from build123d import *

# Parameters (mm, degrees)
BOSS_EXTRUDE1_DEPTH   = 1.57
BOSS_EXTRUDE1_2_DEPTH = 1.57
SKETCH2_W             = 20.9
SKETCH2_H             = 15.9
SKETCH2_W_2           = 94.45
SKETCH2_H_2           = 0.025
SKETCH2_H_3           = 6.025
BOSS_EXTRUDE3_DEPTH   = 6


with BuildPart() as part:
    # Sketch1 → Boss-Extrude1 (new body)
    with BuildSketch(Plane.XY.offset(7.67)):
        with BuildLine():
            Line((-10.2, 60.925), (-45.45, 60.925))
            Line((-45.45, 60.925), (-45.45, 66.925))
            Line((-45.45, 66.925), (45.45, 66.925))
            Line((45.45, 66.925), (45.45, 60.925))
            Line((45.45, 60.925), (10.2, 60.925))
            ThreePointArc((10.2, 60.925), (9.369149532, 61.269149532), (9.025, 62.1))
            Line((9.025, 62.1), (9.025, 63.7))
            ThreePointArc((9.025, 63.7), (8.666205807, 64.566205807), (7.8, 64.925))
            Line((7.8, 64.925), (6.2, 64.925))
            ThreePointArc((6.2, 64.925), (5.333794193, 64.566205807), (4.975, 63.7))
            Line((4.975, 63.7), (4.975, 62.1))
            ThreePointArc((4.975, 62.1), (4.630850468, 61.269149532), (3.8, 60.925))
            Line((3.8, 60.925), (-3.8, 60.925))
            ThreePointArc((-3.8, 60.925), (-4.630850468, 61.269149532), (-4.975, 62.1))
            Line((-4.975, 62.1), (-4.975, 63.7))
            ThreePointArc((-4.975, 63.7), (-5.333794193, 64.566205807), (-6.2, 64.925))
            Line((-6.2, 64.925), (-7.8, 64.925))
            ThreePointArc((-7.8, 64.925), (-8.666205807, 64.566205807), (-9.025, 63.7))
            Line((-9.025, 63.7), (-9.025, 62.1))
            ThreePointArc((-9.025, 62.1), (-9.369149532, 61.269149532), (-10.2, 60.925))
        make_face()
    extrude(amount=-BOSS_EXTRUDE1_DEPTH)



with BuildPart() as body_2:
    # Sketch1 → Boss-Extrude1 2 (new body)
    with BuildSketch(Plane.XY.offset(7.67)):
        with BuildLine():
            Line((10.2, -60.925), (45.45, -60.925))
            Line((45.45, -60.925), (45.45, -66.925))
            Line((45.45, -66.925), (-45.45, -66.925))
            Line((-45.45, -66.925), (-45.45, -60.925))
            Line((-45.45, -60.925), (-10.2, -60.925))
            ThreePointArc((-10.2, -60.925), (-9.369149532, -61.269149532), (-9.025, -62.1))
            Line((-9.025, -62.1), (-9.025, -63.7))
            ThreePointArc((-9.025, -63.7), (-8.666205807, -64.566205807), (-7.8, -64.925))
            Line((-7.8, -64.925), (-6.2, -64.925))
            ThreePointArc((-6.2, -64.925), (-5.333794193, -64.566205807), (-4.975, -63.7))
            Line((-4.975, -63.7), (-4.975, -62.1))
            ThreePointArc((-4.975, -62.1), (-4.630850468, -61.269149532), (-3.8, -60.925))
            Line((-3.8, -60.925), (3.8, -60.925))
            ThreePointArc((3.8, -60.925), (4.630850468, -61.269149532), (4.975, -62.1))
            Line((4.975, -62.1), (4.975, -63.7))
            ThreePointArc((4.975, -63.7), (5.333794193, -64.566205807), (6.2, -64.925))
            Line((6.2, -64.925), (7.8, -64.925))
            ThreePointArc((7.8, -64.925), (8.666205807, -64.566205807), (9.025, -63.7))
            Line((9.025, -63.7), (9.025, -62.1))
            ThreePointArc((9.025, -62.1), (9.369149532, -61.269149532), (10.2, -60.925))
        make_face()
    extrude(amount=-BOSS_EXTRUDE1_2_DEPTH)


with BuildPart() as part_1:
    add(part.part)

    add(body_2.part)  # Boss-Extrude3 merges body 2
    # Sketch2 → Boss-Extrude3 (add)
    with BuildSketch(Plane.XY.offset(0.1)):
        with BuildLine():
            ThreePointArc((-45.621153846, 16.138909297), (-42.65479168, 19.145865857), (-41.280343138, 23.139859279))
            ThreePointArc((-41.280343138, 23.139859279), (-44.331790058, 26.826513587), (-45.425, 31.485659466))
            Line((-45.425, 31.485659466), (-45.45, 66.925))
            Line((-45.45, 66.925), (45.45, 66.925))
            Line((45.45, 66.925), (45.425, 31.485659466))
            ThreePointArc((45.425, 31.485659466), (44.331790058, 26.826513587), (41.280343138, 23.139859279))
            ThreePointArc((41.280343138, 23.139859279), (42.65479168, 19.145865857), (45.621153846, 16.138909297))
            ThreePointArc((45.621153846, 16.138909297), (46.797776617, 14.880036243), (47.225, 13.21070024))
            Line((47.225, 13.21070024), (47.225, 0.025))
            Line((47.225, 0.025), (-47.225, 0.025))
            Line((-47.225, 0.025), (-47.225, 13.21070024))
            ThreePointArc((-47.225, 13.21070024), (-46.797776617, 14.880036243), (-45.621153846, 16.138909297))
        make_face()
        with Locations((0, 52.95)):
            Rectangle(SKETCH2_W, SKETCH2_H, mode=Mode.SUBTRACT)
        with Locations((0, 0.0125)):
            Rectangle(SKETCH2_W_2, SKETCH2_H_2)
        with Locations((0, -0.0125)):
            Rectangle(SKETCH2_W_2, SKETCH2_H_2)
        with BuildLine():
            Line((-47.225, -0.025), (-47.225, -13.21070024))
            ThreePointArc((-47.225, -13.21070024), (-46.797776617, -14.880036243), (-45.621153846, -16.138909297))
            ThreePointArc((-45.621153846, -16.138909297), (-42.65479168, -19.145865857), (-41.280343138, -23.139859279))
            ThreePointArc((-41.280343138, -23.139859279), (-44.331790058, -26.826513587), (-45.425, -31.485659466))
            Line((-45.425, -31.485659466), (-45.45, -66.925))
            Line((-45.45, -66.925), (-30.45, -66.925))
            Line((-30.45, -66.925), (-30.45, -45))
            Line((-30.45, -45), (-10.45, -45))
            Line((-10.45, -45), (10.45, -45))
            Line((10.45, -45), (30.45, -45))
            Line((30.45, -45), (30.45, -66.925))
            Line((30.45, -66.925), (45.45, -66.925))
            Line((45.45, -66.925), (45.425, -31.485659466))
            ThreePointArc((45.425, -31.485659466), (44.331790058, -26.826513587), (41.280343138, -23.139859279))
            ThreePointArc((41.280343138, -23.139859279), (42.65479168, -19.145865857), (45.621153846, -16.138909297))
            ThreePointArc((45.621153846, -16.138909297), (46.797776617, -14.880036243), (47.225, -13.21070024))
            Line((47.225, -13.21070024), (47.225, -0.025))
            Line((47.225, -0.025), (-47.225, -0.025))
        make_face()
        Polygon((10.45, -60.9), (10.45, -66.925), (30.45, -66.925), (30.45, -45), (10.45, -45), align=None)
        Polygon((-30.45, -45), (-30.45, -66.925), (-10.45, -66.925), (-10.45, -60.9), (-10.45, -45), align=None)
        with Locations((0, -63.9125)):
            Rectangle(SKETCH2_W, SKETCH2_H_3)
    extrude(amount=BOSS_EXTRUDE3_DEPTH)


solid = part_1.part
Here's how the part is built. I have some questions about the finished solid (model axes, mm). A direction names the side the tool comes from. Coordinates: 2 decimals unless noted, no trailing zeros. Loops run counter-clockwise (first coordinate to the right, second up) from the corner with the lowest first, then second, coordinate; pieces in that order, holes last. Notation, with made-up numbers: (32.25, 16) -> (44.25, 16) arc R30 ccw to (44.25, 43) -> close; hole circle Ø2 at (-23.5, 35). An arc over 180 degrees is marked (long way). Use one line per item in the form item = value. Start each with the question number.
(1) If we section it at A-A (z = 2.5): Please give me the cut outline in (x, y) (3 decimals), then the cut area to 3 significant figures.
(2) Will these pins go through, and if not, where does the flat tip stop? pin 1 (0.8 mm diameter, centred on y = 62.5, z = 7, fed in from -X); pin 2 (6 mm diameter, centred on x = -19.5, y = -10, fed in from +Z); pin 3 (0.8 mm diameter, centred on y = 63, z = 7, fed in from +X).
(3) If we section it at C-C (x = 29.5): Please give me the cut outline in (y, z) (3 decimals), then the cut area to 3 significant figures.
(4) On a 3-axis mill with a long thin cutter (end or side, diameter ignored), from which of +Z, -Z, +X, -X, +Y, -Y can I reach the whole of each face in a straight line? I mean faces 1 (the face through (1, 64, 7.67)), 2 (the face through (-44.302, 26.766, 3.058)), 3 (the face through (-1, 66.925, 4)), 4 (the face through (44.362, 26.887, 3.058)), 5 (the face through (10.45, 53, 3)). Say none if no direction works.
(5) We'd pull the mould along X, two halves only. Please class faces 6 (the face through (42.62, -19.2, 3.06)), 7 (the face through (0, -45, 3)), 8 (the face through (-46.81, 14.86, 3.06)): pulls with the +X half, pulls with the -X half, needs draft (parallel to the pull), parting line crosses it, or undercut.
(6) If we section it at D-D (y = -2.5): Please give me the cut outline in (x, z) (3 decimals), then the cut area to 3 significant figures.
(7) Please list where these lines run through material, in increasing order: line 1 along X through (y, z) = (59, 4.5); line 2 along Y through (x, z) = (4, 1.5) (3 decimals); line 3 along Y through (x, z) = (28, 6.5) (3 decimals).
(8) If we section it at B-B (y = 52.5): Please give me the cut outline in (x, z), then the cut area to 3 significant figures.
Verdict:
q1.outline = (-47.225, -13.211) arc R3.475 ccw to (-45.621, -16.139) arc R9.525 cw to (-41.28, -23.14) arc R10.475 ccw to (-45.425, -31.486) -> (-45.45, -66.925) -> (45.45, -66.925) -> (45.425, -31.486) arc R10.475 ccw to (41.28, -23.14) arc R9.525 cw to (45.621, -16.139) arc R3.475 ccw to (47.225, -13.211) -> (47.225, 13.211) arc R3.475 ccw to (45.621, 16.139) arc R9.525 cw to (41.28, 23.14) arc R10.475 ccw to (45.425, 31.486) -> (45.45, 66.925) -> (-45.45, 66.925) -> (-45.425, 31.486) arc R10.475 ccw to (-41.28, 23.14) arc R9.525 cw to (-45.621, 16.139) arc R3.475 ccw to (-47.225, 13.211) -> close; hole (-10.45, -60.9) -> (10.45, -60.9) -> (10.45, -45) -> (-10.45, -45) -> close; hole (-10.45, 45) -> (10.45, 45) -> (10.45, 60.9) -> (-10.45, 60.9) -> close
q1.area = 11,500 mm²
q2.pin_1 = -45.45
q2.pin_2 = 6.1
q2.pin_3 = 45.45
q3.outline = (-66.925, 0.1) -> (66.925, 0.1) -> (66.925, 7.67) -> (60.925, 7.67) -> (60.925, 6.1) -> (-60.925, 6.1) -> (-60.925, 7.67) -> (-66.925, 7.67) -> close
q3.area = 822 mm²
q4.face_1 = +Z, +X, -X, +Y, -Y
q4.face_2 = +Z, -Z, -X
q4.face_3 = +Z, -Z, +X, -X, +Y
q4.face_4 = +Z, -Z, +X
q4.face_5 = +Z, -Z
q5.face_6 = pulls with the +X half
q5.face_7 = undercut
q5.face_8 = pulls with the -X half
q6.outline = (-47.225, 0.1) -> (47.225, 0.1) -> (47.225, 6.1) -> (-47.225, 6.1) -> close
q6.area = 567 mm²
q7.line_1 = -45.44 to -10.45, 10.45 to 45.44
q7.line_2 = -66.925 to -60.9, -45 to 45, 60.9 to 66.925
q7.line_3 = -66.925 to -60.925, 60.925 to 66.925
q8.outline = (-45.44, 0.1) -> (-10.45, 0.1) -> (-10.45, 6.1) -> (-45.44, 6.1) -> close; (10.45, 0.1) -> (45.44, 0.1) -> (45.44, 6.1) -> (10.45, 6.1) -> close
q8.area = 420 mm²
